For this review, take the finished solid that the model builds, in its own axes (mm). A direction names the side the tool comes from. Coordinates: 2 decimals unless noted, no trailing zeros. Write each loop counter-clockwise with the first axis right and the second up, starting at its lowest first coordinate (ties: lowest second). Pieces come first, ordered by that corner, then holes. Notation, with made-up numbers: (59.25, 88) - (85.25, 88) arc R15 cw to (85.25, 110) - close; hole circle Ø9 at (68, -25). An arc over 180 degrees is marked (long way). Use one line per item in the form item = value. Start each with the question number.
1) For L1, parallel to Y at x = 29.5, z = -31; L2, parallel to Y at x = -40.5, z = 28; L3, parallel to Z at x = 2, y = 7.5, list the stretches that pass through material, from the lowest coordinate up. Write a range as from..to.
2) We need section B-B (y = 12.5). Give the boundary of the cut face in (x, z), plus the area to 3 significant figures.
3) We need section A-A (x = -11.5). Give the boundary of the cut face in (y, z), plus the area to 3 significant figures.
4) We need section C-C (y = 89). Give the boundary of the cut face in (x, z).
5) We need section D-D (z = 38.5). Give the boundary of the cut face in (x, y), plus the area to 3 significant figures.
6) Insertion check: P1, Ø12, axis at x = -24, y = 8.5, coming from the -Z side; P2, Ø2.5, axis at x = 45.5, y = 56.5, coming from the +Z side; P3, Ø5.5, axis at x = 41.5, y = 56.5, coming from the -Z side. Each pin has a flat end and moves straight along its axis. Give the tip position at first contact, or say it passes through.
7) Tool access review of faces 4 (the flat face through (42, 89, -31.087)), 5 (the flat face through (52.338, 88.535, -36.714)), 6 (the flat face through (32.662, 88.535, -48.286)), 7 (the flat face through (-11, 7, -62.5)): name each direction out of +Z, -Z, +X, -X, +Y, -Y from which nothing blocks a thin tool from reaching the whole face with its end or side.
8) Mouldability with a two-part tool opening along X and no side actions: class faces 1 (the cylindrical face through (8.625, 7.395, 33.126)), 2 (the flat face through (52.43, 88.54, -48.13)), 3 (the flat face through (53, 91, -48)) as pulls with the +X half, pulls with the -X half, needs draft (parallel to the pull), parting line crosses it, or undercut.
Autodesk Inventor part; units mm, degrees
ref_plane "YZ Plane" through (0, 0, 0) normal (1, 0, 0) x (0, 1, 0)
ref_plane "XZ Plane" through (0, 0, 0) normal (0, 1, 0) x (-1, 0, 0)
ref_plane "XY Plane" through (0, 0, 0) normal (0, 0, 1) x (1, 0, 0)
sketch "スケッチ1" plane through (0, 0, 0) normal (0, 1, 0) x (-1, 0, 0)
  line L0 (62.5, -62.5) -> (-42.5, -62.5)
  line L1 (-62.5, -42.5) -> (-62.5, 62.5)
  line L2 (-62.5, 62.5) -> (62.5, 62.5)
  line L3 (62.5, 62.5) -> (62.5, -62.5)
  line L4 (62.5, -62.5) -> (-62.5, 62.5) construction
  line L5 (-62.5, -62.5) -> (62.5, 62.5) construction
  line L6 (17.5, 62.5) -> (62.5, 17.5)
  circle A0 centre (-42.5, -42.5) radius 20
  point P0 (0, 0)
  dimension "d0" = 125
  dimension "d1" = 125
  dimension "d2" = 80
  dimension "d3" = 80
  dimension "d4" = 40
  dimension "d5" = 20
extrude "押し出し1" add sketch "スケッチ1" along normal blind 15 contours L0 A0 L1 L2 L6 L3
extrude "押し出し2" add sketch "スケッチ1" along normal blind 53 contours A0
sketch "スケッチ2" plane through (42.5, 53, -42.5) normal (0, 1, 0) x (1, 0, 0)
  point P0 (-42.5, -42.5)
sketch "スケッチ3" plane through (42.5, 53, -42.5) normal (0, 1, 0) x (1, 0, 0)
  circle A0 centre (0, 0) radius 20
  circle A1 centre (0, 0) radius 7.5
  line L0 (13.1788, 0) -> (6.5894, -11.4132)
  line L1 (6.5894, -11.4132) -> (-6.5894, -11.4132)
  line L2 (-6.5894, -11.4132) -> (-13.1788, 0)
  line L3 (-13.1788, 0) -> (-6.5894, 11.4132)
  line L4 (-6.5894, 11.4132) -> (6.5894, 11.4132)
  line L5 (6.5894, 11.4132) -> (13.1788, 0)
  point P0 (-42.5, -42.5)
  dimension "d10" = 15
extrude "押し出し3" add sketch "スケッチ3" along normal blind 38 contours A1
extrude "押し出し4" add sketch "スケッチ3" along normal blind 5 contours L0 L1 L2 L3 L4 L5
sketch "スケッチ4" plane through (42.5, 91, -42.5) normal (0, 1, 0) x (1, 0, 0)
  circle A0 centre (0, 0) radius 7.5
  line L0 (6.5894, -11.4132) -> (13.1788, 0)
  line L1 (13.1788, 0) -> (6.5894, 11.4132)
  line L2 (6.5894, 11.4132) -> (-6.5894, 11.4132)
  line L3 (-6.5894, 11.4132) -> (-13.1788, 0)
  line L4 (-13.1788, 0) -> (-6.5894, -11.4132)
  line L5 (-6.5894, -11.4132) -> (6.5894, -11.4132)
  circle A1 centre (0, 0) radius 7.5
  point P0 (-42.5, -42.5)
extrude "押し出し5" add sketch "スケッチ4" against normal blind 5
thread "ねじ1"
sketch "スケッチ5" plane through (42.5, 91, -42.5) normal (0, 1, 0) x (1, 0, 0)
  circle A0 centre (0, 0) radius 28
  point P0 (-42.5, -42.5)
  dimension "d19" = 56
extrude "押し出し6" add sketch "スケッチ5" along normal blind 14
fillet "フィレット1" radius 4 1 edges at (14.5, 91, -42.5)
sketch "スケッチ7" plane through (0, 0, 0) normal (0, -1, 0) x (1, 0, 0)
  point P0 (0, 0)
sketch "スケッチ8" plane through (0, 0, 0) normal (0, -1, 0) x (1, 0, 0)
  circle A0 centre (-50.4462, 10.8482) radius 2.5
  line L0 (62.5, -62.5) -> (-62.5, 62.5) construction
  circle A1 centre (-10.8482, 50.4462) radius 2.5
  circle A2 centre (-30.6472, -8.9508) radius 2.5
  line L1 (-50.4462, 10.8482) -> (-10.8482, 50.4462)
  circle A3 centre (8.9508, 30.6472) radius 2.5
  line L2 (-30.6472, -8.9508) -> (8.9508, 30.6472)
  point P0 (0, 0)
  dimension "d23" = 5
  dimension "d24" = 28
  dimension "d25" = 5
  dimension "d26" = 28
  dimension "d27" = 28
extrude "押し出し7" cut sketch "スケッチ8" against normal blind 15
properties part number "foot"
Determined:
q1.L1 = 0..53, 91..105
q1.L2 = 0..15
q1.L3 = -62.5..62.5
q2.outline = (-62.5, -62.5) - (42.5, -62.5) arc R20 ccw to (62.5, -42.5) - (62.5, 62.5) - (-17.5, 62.5) - (-62.5, 17.5) - close; hole circle Ø5 at (-50.45, 10.85); hole circle Ø5 at (-30.65, -8.95); hole circle Ø5 at (-10.85, 50.45); hole circle Ø5 at (8.95, 30.65)
q2.area = 14,400 mm²
q3.outline = (0, -62.5) - (15, -62.5) - (15, 48.03) - (0, 48.03) - close; (0, 52.86) - (15, 52.86) - (15, 62.5) - (0, 62.5) - close
q3.area = 1,800 mm²
q4.outline = (29.32, -42.5) - (35.91, -53.91) - (49.09, -53.91) - (55.68, -42.5) - (49.09, -31.09) - (35.91, -31.09) - close
q5.outline = (-41.5, 0) - (62.5, 0) - (62.5, 15) - (-41.5, 15) - close
q5.area = 1,560 mm²
q6.P1 = -62.5
q6.P2 = -31.09
q6.P3 = -53.91
q7.face_4 = +Z, +X, -X
q7.face_5 = +Z, +X
q7.face_6 = -Z, -X
q7.face_7 = -Z, +X, -X, -Y
q8.face_1 = undercut
q8.face_2 = pulls with the +X half
q8.face_3 = needs draft
